Solid Edge part; units mm, degrees
sketch "Sketch1" plane through (0, 0, 0) normal (0, -1, 0) x (1, 0, 0)
  line L0 (30, 0) -> (30, 29.7921)
  line L1 (30, 29.7921) -> (0, 3.3346)
  line L2 (0, 3.3346) -> (0, 0)
  line L3 (0, 0) -> (30, 0)
extrude "Protrusion1" add sketch "Sketch1" against normal blind 30
shell "Thinwall_1" thickness 3 removed faces 1 at (25.3, 24.7, 25.6471)
hole "Hole_1" at (14.9984, 15, 3) direction (0, 0, -1) diameter 5.0546 end up to next
Build history of the part. All positions in model axes, mm. A direction names the side the tool comes from. Round coordinates to 2 decimals unless told otherwise and drop trailing zeros. Order: outer loops, then holes, each group sorted by start corner. A loop starts at its lowest first (then second) coordinate and runs counter-clockwise, first axis right, second up. Notation, with made-up numbers: (57, -26) -> (78, -26) arc R22 cw to (78, -2) -> close; hole circle Ø7 at (44, 64). An arc over 180 degrees is marked (long way). Answer in a Markdown table with one row per item.
1) Which spindle directions (+Z, -Z, +X, -X, +Y, -Y) get a long thin tool onto all of the face, cutting with end or side? Do faces 1 (the flat face through (12, 15, 3)), 2 (the flat face through (30, 15, 15)). Say none if no direction does.
Values:
| item | result |
|---|---|
| face 1 | +Z |
| face 2 | +Z, -Z, +X, +Y, -Y |
2) Band-saw the part on C-C on x = 13. Give the cut face in (y, z).
Values:
| item | result |
|---|---|
| outline | (0, 0) -> (13.45, 0) -> (13.45, 3) -> (3, 3) -> (3, 14.8) -> (0, 14.8) -> close; (16.55, 0) -> (30, 0) -> (30, 14.8) -> (27, 14.8) -> (27, 3) -> (16.55, 3) -> close |
3) Band-saw the part on A-A on y = 15. Give the cut face in (x, z), and give its area (3 significant figures).
Values:
| item | result |
|---|---|
| outline | (0, 0) -> (12.47, 0) -> (12.47, 3) -> (3, 3) -> (3, 5.98) -> (0, 3.33) -> close; (17.53, 0) -> (30, 0) -> (30, 29.79) -> (27, 27.15) -> (27, 3) -> (17.53, 3) -> close |
| area | 156 mm2 |
4) Mould opens along Y. For faces 3 (the flat face through (15.21, 1.46, 16.75)), 4 (the flat face through (19, 0, 12)), 5 (the flat face through (27, 15, 15)) say: released by +Y, released by -Y, zero draft, split by the parting line, or undercut.
Values:
| item | result |
|---|---|
| face 3 | zero draft |
| face 4 | released by -Y |
| face 5 | undercut |
5) Pin check, flat tips, straight feed: P1, Ø10, axis at x = 13.5, y = 16, coming from the +Z side; P2, Ø2, axis at y = 6.5, z = 18.5, coming from the -X side; P3, Ø4, axis at y = 8, z = 7, coming from the -X side; P4, Ø4, axis at x = 16.5, z = 11, coming from the -Y side. Stop position of each tip, or through.
Values:
| item | result |
|---|---|
| P1 | z = 3 |
| P2 | x = 27 |
| P3 | x = 1.89 |
| P4 | y = 0 |
6) Band-saw the part on B-B on y = 12. Give the cut face in (x, z).
Values:
| item | result |
|---|---|
| outline | (0, 0) -> (30, 0) -> (30, 29.79) -> (27, 27.15) -> (27, 3) -> (3, 3) -> (3, 5.98) -> (0, 3.33) -> close |
7) Wall check: L1, parallel to Y at x = 11, z = 7; L2, parallel to X at y = 15, z = 1.9; L3, parallel to X at y = 10.5, z = 13. Give the ranges that are in metal, low to high.
Values:
| item | result |
|---|---|
| L1 | 0 to 3, 27 to 30 |
| L2 | 0 to 12.47, 17.53 to 30 |
| L3 | 27 to 30 |
8) Band-saw the part on D-D on z = 5.5. Give the cut face in (x, y).
Values:
| item | result |
|---|---|
| outline | (2.46, 0) -> (30, 0) -> (30, 30) -> (2.46, 30) -> close; hole (3, 3) -> (27, 3) -> (27, 27) -> (3, 27) -> close |
